Geometry check sheet. Reference: the model listing, model coordinates, mm. Coordinates: 2 decimals unless noted, no trailing zeros. Loops run counter-clockwise (first coordinate to the right, second up) from the corner with the lowest first, then second, coordinate; pieces in that order, holes last.
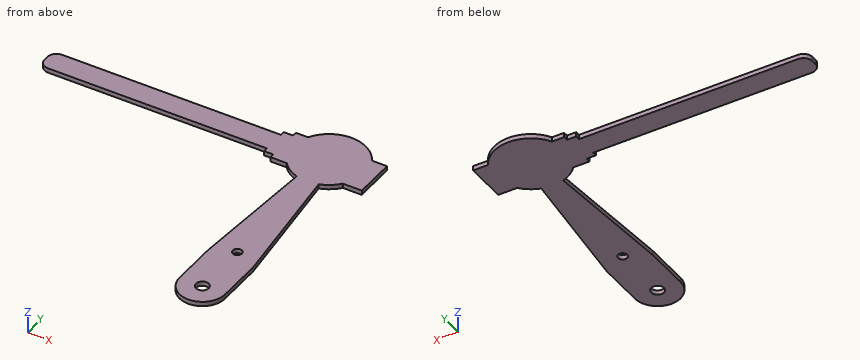
from build123d import *

# Parameters (mm, degrees)
MODEL_R           = 1.4
MODEL_R_2         = 1
BRIDA_BASE1_DEPTH = 1


# Sheet-metal steps are written as plain solids
with BuildPart() as part:
    # Model → Brida base1 (new body)
    with BuildSketch(Plane.XY):
        with BuildLine():
            Line((40.2059904, -5.7615616), (42.197855138, 22.819737764))
            ThreePointArc((42.197855138, 22.819737764), (40.144837503, 23.807467685), (38.45349381, 25.333851753))
            Line((38.45349381, 25.333851753), (34.906389557, 25.333851753))
            Line((34.906389557, 25.333851753), (34.906389557, 26.333851753))
            Line((34.906389557, 26.333851753), (32.906389557, 26.333851753))
            Line((32.906389557, 26.333851753), (32.906389557, 27.333851753))
            Line((32.906389557, 27.333851753), (-15.093610443, 27.333851753))
            ThreePointArc((-15.093610443, 27.333851753), (-16.507824005, 27.919638191), (-17.093610443, 29.333851753))
            Line((-17.093610443, 29.333851753), (-17.093610443, 30.333851753))
            ThreePointArc((-17.093610443, 30.333851753), (-16.507824005, 31.748065316), (-15.093610443, 32.333851753))
            Line((-15.093610443, 32.333851753), (32.906389557, 32.333851753))
            Line((32.906389557, 32.333851753), (32.906389557, 33.333851753))
            Line((32.906389557, 33.333851753), (34.906389557, 33.333851753))
            Line((34.906389557, 33.333851753), (34.906389557, 34.333851753))
            Line((34.906389557, 34.333851753), (37.610831115, 34.333851753))
            ThreePointArc((37.610831115, 34.333851753), (44.604363348, 38.449201588), (51.597895581, 34.333851753))
            Line((51.597895581, 34.333851753), (54.906389557, 34.333851753))
            Line((54.906389557, 34.333851753), (54.906389557, 25.333851753))
            Line((54.906389557, 25.333851753), (50.755232885, 25.333851753))
            ThreePointArc((50.755232885, 25.333851753), (49.063889193, 23.807467685), (47.010871557, 22.819737764))
            Line((47.010871557, 22.819737764), (50.2059904, -5.7615616))
            Line((50.2059904, -5.7615616), (50.2059904, -15.7615616))
            ThreePointArc((50.2059904, -15.7615616), (45.2059904, -20.7615616), (40.2059904, -15.7615616))
            Line((40.2059904, -15.7615616), (40.2059904, -5.7615616))
        make_face()
        with Locations((45.2059904, -15.7615616)):
            Circle(MODEL_R, mode=Mode.SUBTRACT)
        with Locations((45.2059904, -3.2615616)):
            Circle(MODEL_R_2, mode=Mode.SUBTRACT)
    extrude(amount=-BRIDA_BASE1_DEPTH)


solid = part.part
1) Section check A-A on x = 48. Record the cut outline in (y, z), and give its area (3 significant figures).
Data:
outline: (-19.91, -1) - (13.97, -1) - (13.97, 0) - (-19.91, 0) - close; (23.21, -1) - (37.69, -1) - (37.69, 0) - (23.21, 0) - close
area: 48.4 mm2
2) Material ranges on probe 1 along Y at (x, z) = (46, -0.6); probe 2 along Y at (x, z) = (-5, -0.2); probe 3 along X at (y, z) = (26, -0.9), recorded low to high.
Data:
probe 1: y = -20.7 to -16.91, -14.61 to -3.87, -2.65 to 38.33
probe 2: y = 27.33 to 32.33
probe 3: x = 34.91 to 54.91
3) Depth check by flat-ended pin: pin 1 (0.5 mm diameter, centred on y = 26, z = -0.5, fed in from -X); pin 2 (0.5 mm diameter, centred on x = 12.5, z = -0.5, fed in from +Y); pin 3 (0.5 mm diameter, centred on x = 52.5, z = -0.5, fed in from +Y). Enter the tip coordinate at first touch or a pass-through.
Data:
pin 1: stops at x = 34.91
pin 2: stops at y = 32.33
pin 3: stops at y = 34.33
4) Section check B-B on z = -0.2. Record the cut outline in (x, y).
Data:
outline: (-17.09, 29.33) arc R2 ccw to (-15.09, 27.33) - (32.91, 27.33) - (32.91, 26.33) - (34.91, 26.33) - (34.91, 25.33) - (38.45, 25.33) arc R8 ccw to (42.2, 22.82) - (40.21, -5.76) - (40.21, -15.76) arc R5 ccw to (50.21, -15.76) - (50.21, -5.76) - (47.01, 22.82) arc R8 ccw to (50.76, 25.33) - (54.91, 25.33) - (54.91, 34.33) - (51.6, 34.33) arc R8 ccw to (37.61, 34.33) - (34.91, 34.33) - (34.91, 33.33) - (32.91, 33.33) - (32.91, 32.33) - (-15.09, 32.33) arc R2 ccw to (-17.09, 30.33) - close; hole circle Ø2.8 at (45.21, -15.76); hole circle Ø2 at (45.21, -3.26)
5) Section check D-D on x = -3. Record the cut outline in (y, z).
Data:
outline: (27.33, -1) - (32.33, -1) - (32.33, 0) - (27.33, 0) - close
6) Section check C-C on y = -10.5. Record the cut outline in (x, z).
Data:
outline: (40.21, -1) - (50.21, -1) - (50.21, 0) - (40.21, 0) - close
